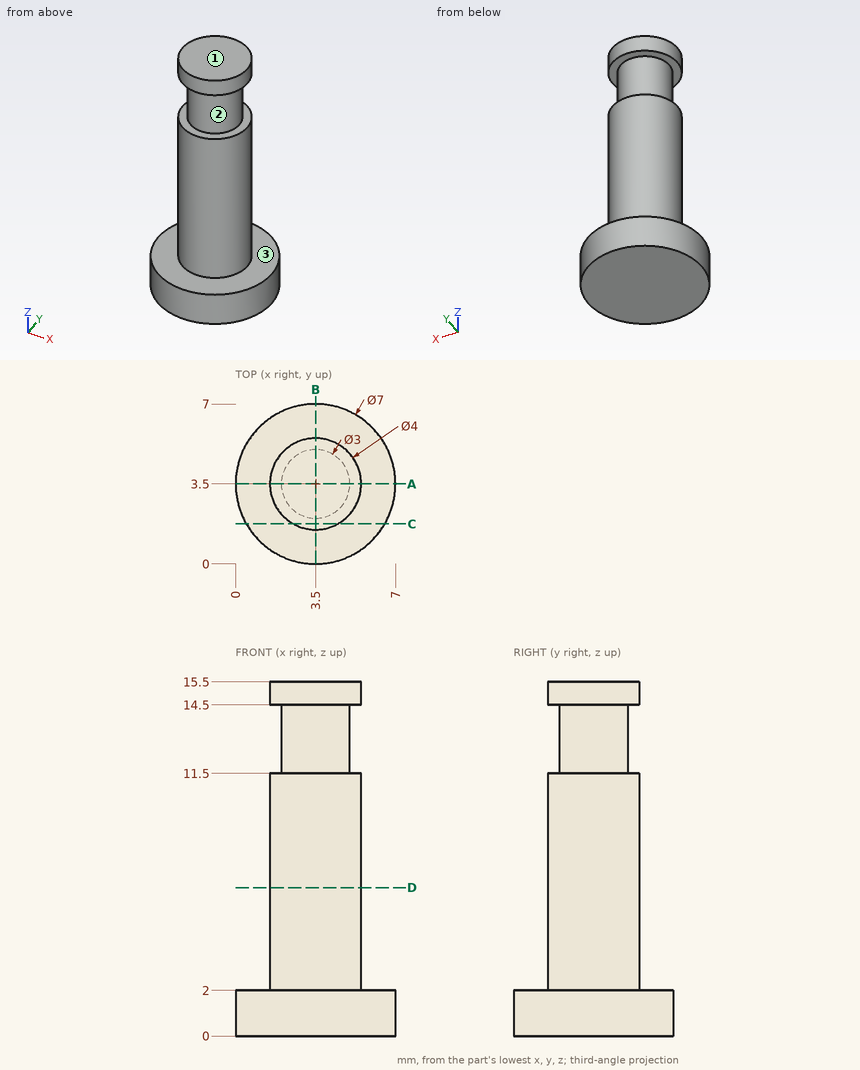
Answer from the drawing. Dimensions are ordinates in mm from the lowest x, y and z of the part. A direction names the side the tool comes from. Round coordinates to 2 decimals unless told otherwise and drop trailing zeros. Loops run counter-clockwise (first coordinate to the right, second up) from the corner with the lowest first, then second, coordinate; pieces in that order, holes last.
1) Consider line 1 (Z direction, x = 2.5, y = 2.25); line 2 (Z direction, x = 4.75, y = 6); line 3 (Y direction, x = 3, z = 10). Determine where each line is inside the solid, lowest interval first.
Outcome:
line 1: z = 0 to 11.5, 14.5 to 15.5
line 2: z = 0 to 2
line 3: y = 1.56 to 5.44
2) A cutting plane is placed at C-C on y = 1.75. Determine the outline of the cut face in (x, z), plus the area to 3 significant figures.
Outcome:
outline: (0.47, 0) - (6.53, 0) - (6.53, 2) - (4.47, 2) - (4.47, 11.5) - (2.53, 11.5) - (2.53, 2) - (0.47, 2) - close; (2.53, 14.5) - (4.47, 14.5) - (4.47, 15.5) - (2.53, 15.5) - close
area: 32.5 mm2
3) A cutting plane is placed at A-A on y = 3.5. Determine the outline of the cut face in (x, z).
Outcome:
outline: (0, 0) - (7, 0) - (7, 2) - (5.5, 2) - (5.5, 11.5) - (5, 11.5) - (5, 14.5) - (5.5, 14.5) - (5.5, 15.5) - (1.5, 15.5) - (1.5, 14.5) - (2, 14.5) - (2, 11.5) - (1.5, 11.5) - (1.5, 2) - (0, 2) - close
4) Given P1, Ø4, axis at x = 3, z = 4.5, coming from the -Y side; P2, Ø1.2, axis at x = 3, y = 4, coming from the -Z side; P3, Ø1.5, axis at y = 2.5, z = 12, coming from the +X side; P4, Ø3, axis at x = 1.5, z = 13, coming from the -Y side, each flat-ended and moving along its own axis, determine where each tip first touches the part or whether it passes through.
Outcome:
P1: stops at y = 1.5
P2: stops at z = 0
P3: stops at x = 5.45
P4: stops at y = 2.09
5) For the marked faces 1, 2 and 3, determine the directions among +Z, -Z, +X, -X, +Y, -Y from which every point of the face is accessible in a straight line to the end or side of a thin tool.
Outcome:
face 1: +Z, +X, -X, +Y, -Y
face 2: none
face 3: +Z
6) A cutting plane is placed at D-D on z = 6.5. Determine the outline of the cut face in (x, y), plus the area to 3 significant figures.
Outcome:
outline: circle Ø4 at (3.5, 3.5)
area: 12.6 mm2
